Autodesk Inventor part; units mm, degrees
ref_plane "YZ Plane" through (0, 0, 0) normal (1, 0, 0) x (0, 1, 0)
ref_plane "XZ Plane" through (0, 0, 0) normal (0, 1, 0) x (-1, 0, 0)
ref_plane "XY Plane" through (0, 0, 0) normal (0, 0, 1) x (1, 0, 0)
sketch "Szkic1" plane through (0, 0, 0) normal (0, 1, 0) x (-1, 0, 0)
  line L0 (11.2175, 30.7175) -> (-11.2175, 30.7175)
  line L1 (-11.2175, 30.7175) -> (-11.2175, -30.7175)
  line L2 (11.2175, -30.7175) -> (11.2175, 30.7175)
  circle A0 centre (6.7175, 12.7825) radius 1.5
  circle A1 centre (-6.7175, 26.2175) radius 1.5
  circle A2 centre (0, 19.5) radius 4.5
  circle A3 centre (0, -19.5) radius 4.5
  circle A4 centre (6.7175, -12.7825) radius 1.5
  circle A5 centre (-6.7175, -26.2175) radius 1.5
  circle A6 centre (5.6569, 25.1569) radius 1.5
  circle A7 centre (-5.6569, 13.8431) radius 1.5
  circle A8 centre (-5.6569, -13.8431) radius 1.5
  circle A9 centre (5.6569, -25.1569) radius 1.5
  line L3 (11.2175, -30.7175) -> (-11.2175, -30.7175)
  point P0 (0, 0)
  point P1 (0, 10.7072)
  dimension "d0" = 3
  dimension "d1" = 3
  dimension "d3" = 0
  dimension "d8" = 9
  dimension "d10" = 9
  dimension "d11" = 3
  dimension "d12" = 3
  dimension "d20" = 19.5
  dimension "d21" = 39
  dimension "d26" = 3
  dimension "d27" = 3
  dimension "d28" = 3
  dimension "d29" = 3
  dimension "d30" = 6.7175
  dimension "d31" = 6.7175
  dimension "d32" = 6.7175
  dimension "d33" = 6.7175
  dimension "d34" = 6.7175
  dimension "d35" = 6.7175
  dimension "d36" = 6.7175
  dimension "d37" = 6.7175
  dimension "d38" = 5.6569
  dimension "d39" = 5.6569
  dimension "d40" = 5.6569
  dimension "d41" = 5.6569
  dimension "d42" = 5.6569
  dimension "d43" = 5.6569
  dimension "d44" = 5.6569
  dimension "d45" = 5.6569
  dimension "d48" = 4.5
  dimension "d50" = 4.5
  dimension "d51" = 4.5
  dimension "d52" = 4.5
extrude "Wyciągnięcie proste1" add sketch "Szkic1" along normal blind 2
properties part number "HolderV2"
Here's how the part is built. I have some questions about the finished solid (model axes, mm). Coordinates: 2 decimals unless noted, no trailing zeros. Order: outer loops, then holes, each group sorted by start corner. A loop starts at its lowest first (then second) coordinate and runs counter-clockwise, first axis right, second up. Notation, with made-up numbers: M -14,-19.75 L 9,-19.75 A13 ccw 9,3.25 Z; hole C -5,-1.5 d8. An arc over 180 degrees is marked long. Answer as a JSON object with one key per item and string values. Group by question number.
(1) For pin 1 (11.5 mm diameter, centred on x = 0, z = 19.5, fed in from +Y), with a flat end and sliding along its axis, tell me the tip position at first contact or that it passes through.
(2) Suppose I cut it at A-A, the plane x = 0. Please give me the cut outline in (y, z).
(3) If we mould it in two halves opening along X, with no side actions, what happens to faces 1 (the face through (0, 1, 30.718)), 2 (the face through (-11.218, 1, 0)), 3 (the face through (5.911, 0.986, 24.953)), 4 (the face through (11.218, 1, 0))? For each: released by +X, released by -X, zero draft, split by the parting line, or undercut.
(4) Suppose I cut it at D-D, the plane x = -6. Please give me the cut outline in (y, z).
(5) Suppose I cut it at C-C, the plane y = 1.6. State how many separate pieces and enclosed holes the cut face has, then the cut area to 3 significant figures.
(6) I need wall thicknesses on probe 1 along Z at (x, y) = (0, 1.3); probe 2 along Z at (x, y) = (3, 0.3); probe 3 along X at (y, z) = (0.4, -16.5). Which ranges of each line are inside material? Lowest first, please.
(7) Suppose I cut it at B-B, the plane z = 19.5. Please give me the cut outline in (x, y), then the cut area to 3 significant figures.
Values found:
{
 "1": {"pin 1": "stops at y = 2"},
 "2": {"outline": "M 0,-30.72 L 2,-30.72 L 2,-24 L 0,-24 Z; M 0,-15 L 2,-15 L 2,15 L 0,15 Z; M 0,24 L 2,24 L 2,30.72 L 0,30.72 Z"},
 "3": {"face 1": "zero draft", "face 2": "released by -X", "face 3": "undercut", "face 4": "released by +X"},
 "4": {"outline": "M 0,-30.72 L 2,-30.72 L 2,-26.62 L 0,-26.62 Z; M 0,-23.7 L 2,-23.7 L 2,-14.1 L 0,-14.1 Z; M 0,-11.47 L 2,-11.47 L 2,11.47 L 0,11.47 Z; M 0,14.1 L 2,14.1 L 2,23.7 L 0,23.7 Z; M 0,26.62 L 2,26.62 L 2,30.72 L 0,30.72 Z"},
 "5": {"separate pieces": "1", "enclosed holes": "10", "area": "1,190 mm^2"},
 "6": {"probe 1": "z = -30.72 to -24, -15 to 15, 24 to 30.72", "probe 2": "z = -30.72 to -22.85, -16.15 to 16.15, 22.85 to 30.72", "probe 3": "x = -11.22 to -3.35, 3.35 to 11.22"},
 "7": {"outline": "M -11.22,0 L -4.5,0 L -4.5,2 L -11.22,2 Z; M 4.5,0 L 11.22,0 L 11.22,2 L 4.5,2 Z", "area": "26.9 mm^2"}
}
